Could you check a few things on this model? Use its own coordinates, in mm. A direction names the side the tool comes from. Give positions to 0.01 mm unless a question says otherwise; leave off trailing zeros. Loops run counter-clockwise (first coordinate to the right, second up) from the corner with the lowest first, then second, coordinate; pieces in that order, holes last. Notation, with made-up numbers: (-22.5, 71) - (10.5, 71) arc R11 ccw to (10.5, 86) - close; hole circle Ø1 at (35, 26). An arc over 180 degrees is marked (long way). One line per item, written item: value. Start each with the question number.
Q1. I want a section at A-A (y = -22.75). Please give me the cut outline in (x, z), then the cut area to 3 significant figures.
Q2. If I drill on line 1 (Y direction, x = 2.5, z = 2.5); line 2 (X direction, y = -24.75, z = -0.75); line 3 (Z direction, x = 60, y = -27.75), over which ranges is the centre line in solid material (lowest first)? Write a range as from..to.
Q3. I want a section at D-D (y = -16.25). Please give me the cut outline in (x, z).
Q4. I'm going to push flat-ended pins straight in: P1, Ø1, axis at x = 9, y = -13.5, coming from the +Z side; P2, Ø1.5, axis at y = -5.5, z = 2.5, coming from the +X side; P3, Ø1, axis at y = -15, z = -2.5, coming from the +X side. Where does each tip first touch, or does it pass through?
Q5. I want a section at B-B (z = -1). Count the separate pieces of the cut face and the enclosed holes in it, then the cut area to 3 significant figures.
Q6. If we mould it in two halves opening along Y, with no side actions, what happens to faces 1 (the face through (30, 0, -3)), 2 (the face through (54.736, -15, -3)), 3 (the face through (29, -15, -4))? For each: released by +Y, released by -Y, zero draft, split by the parting line, or undercut.
Q7. I want a section at C-C (x = 8.5). Please give me the cut outline in (y, z), then the cut area to 3 significant figures.
Q8. For faces 4 (the face through (2, -20, -2)), 5 (the face through (30, -30, -3)), 6 (the face through (58, -10, -2)), which set-ups out of +Z, -Z, +X, -X, +Y, -Y let a thin tool reach every point of the face, with its end or its side?
```python
from build123d import *

# Parameters (mm, degrees)
F1_DEPTH = 30
F2_W     = 5
F2_H     = 10
F3_DEPTH = 25
F2_W_2   = 4
F4_DEPTH = 25


with BuildPart() as f1:
    # F0 (on Front) → F1 (new body)
    with BuildSketch(Plane.XZ):
        with BuildLine():
            Line((0, -2), (0, -4))
            ThreePointArc((0, -4), (2, -3.4641016151), (3.4641016151, -2))
            Line((3.4641016151, -2), (0, -2))
        make_face()
        with BuildLine():
            ThreePointArc((3.4641016151, -2), (2, -3.4641016151), (0, -4))
            Line((0, -4), (59.7362193561, -4))
            ThreePointArc((59.7362193561, -4), (57.8825422961, -3.4022855387), (56.5308853543, -2))
            Line((56.5308853543, -2), (3.4641016151, -2))
        make_face()
        with BuildLine():
            ThreePointArc((56.5308853543, -2), (57.8825422961, -3.4022855387), (59.7362193561, -4))
            Line((59.7362193561, -4), (60, -4))
            Line((60, -4), (60, -2))
            Line((60, -2), (56.5308853543, -2))
        make_face()
        with BuildLine():
            Line((60, -4), (59.7362193561, -4))
            ThreePointArc((59.7362193561, -4), (62.7335757758, -2.9289055908), (63.9999993682, -0.0087069633))
            ThreePointArc((63.9999993682, -0.0087069633), (58.9695761678, 3.8562934285), (56.5308853543, -2))
            Line((56.5308853543, -2), (60, -2))
            Line((60, -2), (60, -4))
        make_face()
        with BuildLine():
            ThreePointArc((62, 0), (61.4142135624, -1.4142135624), (60, -2))
            ThreePointArc((60, -2), (58.5857864376, 1.4142135624), (62, 0))
        make_face(mode=Mode.SUBTRACT)
        with BuildLine():
            ThreePointArc((3.4641016151, -2), (3.8637033052, -1.0352761804), (4, 0))
            ThreePointArc((4, 0), (-2.8284271247, 2.8284271247), (0, -4))
            Line((0, -4), (0, -2))
            Line((0, -2), (3.4641016151, -2))
        make_face()
        with BuildLine():
            ThreePointArc((2, 0), (1.4142135624, -1.4142135624), (0, -2))
            ThreePointArc((0, -2), (-1.4142135624, 1.4142135624), (2, 0))
        make_face(mode=Mode.SUBTRACT)
    extrude(amount=F1_DEPTH)

    # F2 (on face) → F3 (cut, symmetric)
    with BuildSketch(Plane(origin=(0, 0, -4), x_dir=(1, 0, 0), z_dir=(0, 0, -1))):
        with Locations((57.2362193561, 15)):
            Rectangle(F2_W, F2_H)
        with Locations((62.2362193561, 15)):
            Rectangle(F2_W, F2_H)
    extrude(amount=F3_DEPTH, both=True, mode=Mode.SUBTRACT)

    # F2 (on face) → F4 (cut, symmetric)
    with BuildSketch(Plane(origin=(0, 0, -4), x_dir=(1, 0, 0), z_dir=(0, 0, -1))):
        with Locations((-2, 15)):
            Rectangle(F2_W_2, F2_H)
        with Locations((2.5, 15)):
            Rectangle(F2_W, F2_H)
    extrude(amount=F4_DEPTH, both=True, mode=Mode.SUBTRACT)


solid = f1.part
```
Worked answers:
1. outline: (0, -4) - (59.74, -4) arc R4 ccw (long way) to (56.53, -2) - (3.46, -2) arc R4 ccw (long way) to start; hole circle Ø4 at (0, 0); hole circle Ø4 at (60, 0)
1. area: 186 mm²
2. line 1: y = -30..-20, -10..0
2. line 2: x = -3.93..-1.85, 1.85..3.93, 56.07..58.15, 61.85..63.93
2. line 3: z = -4.01..-2, 2..3.99
3. outline: (5, -4) - (54.74, -4) - (54.74, -2) - (5, -2) - close
4. P1: stops at z = -2
4. P2: stops at x = 63.59
4. P3: stops at x = 54.74
5. separate pieces: 8
5. enclosed holes: 0
5. area: 171 mm²
6. face 1: released by +Y
6. face 2: undercut
6. face 3: zero draft
7. outline: (-30, -4) - (0, -4) - (0, -2) - (-30, -2) - close
7. area: 60.0 mm²
8. face 4: +Z, -Z, -X
8. face 5: +Z, -Z, +X, -X, -Y
8. face 6: +Z, -Z, +X
